Source: CAD feature listing. Evaluate the final solid. Frame: model axes, mm. A direction names the side the tool comes from. Coordinates: 2 decimals unless noted, no trailing zeros. Loops run counter-clockwise (first coordinate to the right, second up) from the corner with the lowest first, then second, coordinate; pieces in that order, holes last.
from build123d import *

# Parameters (mm, degrees)
SKETCH1_W           = 62.15
SKETCH1_H           = 62.15
BOSS_EXTRUDE1_DEPTH = 5
SKETCH3_R           = 31.075
BOSS_EXTRUDE2_DEPTH = 17.7
SKETCH4_R           = 28.575
CUT_EXTRUDE2_DEPTH  = 17.7
BOSS_EXTRUDE3_START = 2.5
SKETCH5_R           = 28.575
SKETCH5_R_2         = 26.075
BOSS_EXTRUDE3_DEPTH = 2.5
CUT_EXTRUDE4_REACH  = 49.377
SKETCH8_R           = 1.5
BOSS_EXTRUDE5_START = 17.7
SKETCH9_R           = 3
SKETCH9_R_2         = 1.5
BOSS_EXTRUDE5_DEPTH = 17.7


with BuildPart() as part:
    # Sketch1 → Boss-Extrude1 (new body)
    with BuildSketch(Plane(origin=(0, 0, 0), x_dir=(1, 0, 0), z_dir=(0, 1, 0))):
        Rectangle(SKETCH1_W, SKETCH1_H)
    extrude(amount=BOSS_EXTRUDE1_DEPTH)

    # Sketch3 → Boss-Extrude2 (add)
    with BuildSketch(Plane(origin=(0, 5, 0), x_dir=(1, 0, 0), z_dir=(0, 1, 0))):
        with Locations(Location((0, 0, 0), (0, 0, 270))):
            Circle(SKETCH3_R)
    extrude(amount=BOSS_EXTRUDE2_DEPTH)

    # Sketch4 → Cut-Extrude2 (cut)
    with BuildSketch(Plane(origin=(0, 22.7, 0), x_dir=(1, 0, 0), z_dir=(0, 1, 0))):
        with Locations(Location((0, 0, 0), (0, 0, 270))):
            Circle(SKETCH4_R)
    extrude(amount=-CUT_EXTRUDE2_DEPTH, mode=Mode.SUBTRACT)

    # Sketch5 → Boss-Extrude3 (add)
    with BuildSketch(Plane(origin=(0, 5, 0), x_dir=(1, 0, 0), z_dir=(0, 1, 0)).offset(BOSS_EXTRUDE3_START)):
        with Locations(Location((0, 0, 0), (0, 0, 270))):
            Circle(SKETCH5_R)
        with Locations(Location((0, 0, 0), (0, 0, 270))):
            Circle(SKETCH5_R_2, mode=Mode.SUBTRACT)
    extrude(amount=-BOSS_EXTRUDE3_DEPTH)

    # Sketch8 → Cut-Extrude4 (cut, up to next)
    with BuildSketch(Plane(origin=(0, 5, 0), x_dir=(1, 0, 0), z_dir=(0, 1, 0)), mode=Mode.PRIVATE) as cut_extrude4_sk1:
        with Locations(Location((-26.075, 26.075, 0), (0, 0, 270))):
            Circle(SKETCH8_R)
    cut_extrude4_tool1 = extrude(cut_extrude4_sk1.sketch, amount=-CUT_EXTRUDE4_REACH, mode=Mode.PRIVATE) & part.part
    # Sketch8 → Cut-Extrude4 (cut, up to next)
    with BuildSketch(Plane(origin=(0, 5, 0), x_dir=(1, 0, 0), z_dir=(0, 1, 0)), mode=Mode.PRIVATE) as cut_extrude4_sk2:
        with Locations(Location((-26.075, -26.075, 0), (0, 0, 270))):
            Circle(SKETCH8_R)
    cut_extrude4_tool2 = extrude(cut_extrude4_sk2.sketch, amount=-CUT_EXTRUDE4_REACH, mode=Mode.PRIVATE) & part.part
    # Sketch8 → Cut-Extrude4 (cut, up to next)
    with BuildSketch(Plane(origin=(0, 5, 0), x_dir=(1, 0, 0), z_dir=(0, 1, 0)), mode=Mode.PRIVATE) as cut_extrude4_sk3:
        with Locations(Location((26.075, -26.075, 0), (0, 0, 270))):
            Circle(SKETCH8_R)
    cut_extrude4_tool3 = extrude(cut_extrude4_sk3.sketch, amount=-CUT_EXTRUDE4_REACH, mode=Mode.PRIVATE) & part.part
    # Sketch8 → Cut-Extrude4 (cut, up to next)
    with BuildSketch(Plane(origin=(0, 5, 0), x_dir=(1, 0, 0), z_dir=(0, 1, 0)), mode=Mode.PRIVATE) as cut_extrude4_sk4:
        with Locations(Location((26.075, 26.075, 0), (0, 0, 270))):
            Circle(SKETCH8_R)
    cut_extrude4_tool4 = extrude(cut_extrude4_sk4.sketch, amount=-CUT_EXTRUDE4_REACH, mode=Mode.PRIVATE) & part.part
    add(cut_extrude4_tool1.solids().sort_by_distance((-26.075, 5, -26.075))[0], mode=Mode.SUBTRACT)
    add(cut_extrude4_tool2.solids().sort_by_distance((-26.075, 5, 26.075))[0], mode=Mode.SUBTRACT)
    add(cut_extrude4_tool3.solids().sort_by_distance((26.075, 5, 26.075))[0], mode=Mode.SUBTRACT)
    add(cut_extrude4_tool4.solids().sort_by_distance((26.075, 5, -26.075))[0], mode=Mode.SUBTRACT)

    # Sketch9 → Boss-Extrude5 (add)
    # profile 1 of 4: a face of its own
    with BuildSketch(Plane(origin=(0, 5, 0), x_dir=(1, 0, 0), z_dir=(0, 1, 0)).offset(BOSS_EXTRUDE5_START)):
        with Locations(Location((-26.075, 26.075, 0), (0, 0, 270))):
            Circle(SKETCH9_R)
        with Locations(Location((-26.075, 26.075, 0), (0, 0, 270))):
            Circle(SKETCH9_R_2, mode=Mode.SUBTRACT)
    # profile 2 of 4: a face of its own
    with BuildSketch(Plane(origin=(0, 5, 0), x_dir=(1, 0, 0), z_dir=(0, 1, 0)).offset(BOSS_EXTRUDE5_START)):
        with Locations(Location((-26.075, -26.075, 0), (0, 0, 90))):
            Circle(SKETCH9_R)
        with Locations(Location((-26.075, -26.075, 0), (0, 0, 270))):
            Circle(SKETCH9_R_2, mode=Mode.SUBTRACT)
    # profile 3 of 4: a face of its own
    with BuildSketch(Plane(origin=(0, 5, 0), x_dir=(1, 0, 0), z_dir=(0, 1, 0)).offset(BOSS_EXTRUDE5_START)):
        with Locations(Location((26.075, -26.075, 0), (0, 0, 270))):
            Circle(SKETCH9_R)
        with Locations(Location((26.075, -26.075, 0), (0, 0, 270))):
            Circle(SKETCH9_R_2, mode=Mode.SUBTRACT)
    # profile 4 of 4: a face of its own
    with BuildSketch(Plane(origin=(0, 5, 0), x_dir=(1, 0, 0), z_dir=(0, 1, 0)).offset(BOSS_EXTRUDE5_START)):
        with Locations(Location((26.075, 26.075, 0), (0, 0, 90))):
            Circle(SKETCH9_R)
        with Locations(Location((26.075, 26.075, 0), (0, 0, 270))):
            Circle(SKETCH9_R_2, mode=Mode.SUBTRACT)
    extrude(amount=-BOSS_EXTRUDE5_DEPTH)


solid = part.part
Q1. Section A-A, the plane y = 19.5. Count the separate pieces of the cut face and the enclosed holes in it, plus the area to 3 significant figures.
Q2. Line query: line 1 along X through (y, z) = (17.5, 0) (3 decimals); line 2 along X through (y, z) = (5.25, 27); line 3 along Z through (x, y) = (-0.5, 16.25). Output: solid intervals per line, ascending.
Q3. Section C-C, the plane z = -22. Return the cut outline in (x, y) (3 decimals), plus the area to 3 significant figures.
Q4. Section B-B, the plane x = -18. Return the cut outline in (y, z) (3 decimals).
Q5. Contact query for flat-ended pins moving along their axis: pin 1 Ø3 at (y, z) = (19, -17.5) entering from -X; pin 2 Ø15.5 at (x, z) = (-10, 15.5) entering from +Y; pin 3 Ø6 at (x, y) = (-5, 15) entering from +Z. Output: stop coordinate, or through.
Q6. Access query for faces 1 (the flat face through (-27.4, 22.7, -24.8)), 2 (the flat face through (-23.7, 5, 23.5)). Directions: +Z, -Z, +X, -X, +Y, -Y. A direction counts if a zero-diameter tool reaches every point of the face in a straight line with its end or side. Return the directions, or none.
Derived:
1. separate pieces: 5
1. enclosed holes: 5
1. area: 553 mm2
2. line 1: x = -31.075 to -28.575, 28.575 to 31.075
2. line 2: x = -28.93 to -27.26, -24.89 to -23.22, -15.38 to 15.38, 23.22 to 24.89, 27.26 to 28.93
2. line 3: z = -31.07 to -28.57, 28.57 to 31.07
3. outline: (-31.075, 0) - (31.075, 0) - (31.075, 5) - (21.947, 5) - (21.947, 22.7) - (18.235, 22.7) - (18.235, 7.5) - (13.997, 7.5) - (13.997, 5) - (-13.997, 5) - (-13.997, 7.5) - (-18.235, 7.5) - (-18.235, 22.7) - (-21.947, 22.7) - (-21.947, 5) - (-31.075, 5) - close
3. area: 463 mm2
4. outline: (0, -31.075) - (5, -31.075) - (5, -25.331) - (22.7, -25.331) - (22.7, -22.193) - (7.5, -22.193) - (7.5, -18.865) - (5, -18.865) - (5, 18.865) - (7.5, 18.865) - (7.5, 22.193) - (22.7, 22.193) - (22.7, 25.331) - (5, 25.331) - (5, 31.075) - (0, 31.075) - close
5. pin 1: stops at x = -26.64
5. pin 2: stops at y = 7.5
5. pin 3: stops at z = 31.01
6. face 1: +Z, -Z, +X, -X, +Y
6. face 2: +Y
